```python
from build123d import *

# Parameters (mm, degrees)
F1_DEPTH = 3


with BuildPart() as f1:
    # F0 (on Front) → F1 (new body)
    with BuildSketch(Plane.XZ):
        with BuildLine():
            Line((-2, 0), (0, 0))
            Line((0, 0), (2, 0))
            Line((2, 0), (2, -3))
            Line((2, -3), (8, -3))
            Line((8, -3), (8, 0))
            Line((8, 0), (12, 0))
            Line((12, 0), (12, 30))
            ThreePointArc((12, 30), (8.485281, 38.485281), (0, 42))
            ThreePointArc((0, 42), (-8.485281, 38.485281), (-12, 30))
            Line((-12, 30), (-12, 0))
            Line((-12, 0), (-8, 0))
            Line((-8, 0), (-8, -3))
            Line((-8, -3), (-2, -3))
            Line((-2, -3), (-2, 0))
        make_face()
        with BuildLine():
            ThreePointArc((0, 23.2), (-6.8, 30), (0, 36.8))
            ThreePointArc((0, 36.8), (6.8, 30), (0, 23.2))
        make_face(mode=Mode.SUBTRACT)
    extrude(amount=F1_DEPTH)


solid = f1.part
```
Verification items for the finished model (mm, model axes). A direction names the side the tool comes from. Give positions to 0.01 mm unless a question says otherwise; leave off trailing zeros. Loops run counter-clockwise (first coordinate to the right, second up) from the corner with the lowest first, then second, coordinate; pieces in that order, holes last. Notation, with made-up numbers: M -33,-32 L -3,-32 A30 ccw -3,-2 Z; hole C 82.25,36.25 d7. An arc over 180 degrees is marked long. One line per question, with ' | ' between items.
Item 1: Tool access check on faces 1 (the face through (-10, -1, 0)), 2 (the face through (2, -1, -1)), 3 (the face through (8, -1, -2)). Record the directions out of +Z, -Z, +X, -X, +Y, -Y that give a thin tool (end or side, any length) a straight path to the whole face; none if there is none.
Completed:
face 1: -Z, -X, +Y, -Y | face 2: -Z, +Y, -Y | face 3: -Z, +X, +Y, -Y
Item 2: Section check A-A, the plane z = 32. Record the cut outline in (x, y).
Completed:
outline: M -11.83,-3 L -6.5,-3 L -6.5,0 L -11.83,0 Z; M 6.5,-3 L 11.83,-3 L 11.83,0 L 6.5,0 Z
Item 3: Section check C-C, the plane y = -2.05. Record the cut outline in (x, z).
Completed:
outline: M -12,0 L -8,0 L -8,-3 L -2,-3 L -2,0 L 2,0 L 2,-3 L 8,-3 L 8,0 L 12,0 L 12,30 A12 ccw 0,42 A12 ccw -12,30 Z; hole C 0,30 d13.6
Item 4: Section check D-D, the plane x = -7.5. Record the cut outline in (y, z).
Completed:
outline: M -3,-3 L 0,-3 L 0,39.37 L -3,39.37 Z
Item 5: Section check B-B, the plane x = 4.25. Record the cut outline in (y, z), plus the area to 3 significant figures.
Completed:
outline: M -3,-3 L 0,-3 L 0,24.69 L -3,24.69 Z; M -3,35.31 L 0,35.31 L 0,41.22 L -3,41.22 Z | area: 101 mm^2
Item 6: Depth check by flat-ended pin: P1, Ø1.5, axis at x = 1, y = -1.5, coming from the -Z side; P2, Ø1.5, axis at y = -1.5, z = -1.5, coming from the +X side; P3, Ø1, axis at y = -1.5, z = 33, coming from the -X side; P4, Ø4, axis at x = 5, z = 28.5, coming from the -Y side. Enter the tip coordinate at first touch or a pass-through.
Completed:
P1: stops at z = 0 | P2: stops at x = 8 | P3: stops at x = -11.74 | P4: stops at y = -3
Item 7: Thickness scan on line 1 (X direction, y = -1.5, z = 30); line 2 (X direction, y = -2.35, z = 33.5); line 3 (Z direction, x = 1, y = -1.2). Record the ranges inside material, lowest first. Write a range as [from, to].
Completed:
line 1: x = [-12, -6.8], [6.8, 12] | line 2: x = [-11.48, -5.83], [5.83, 11.48] | line 3: z = [0, 23.27], [36.73, 41.96]
Item 8: Draft check along X on faces 4 (the face through (-12, -1, 15)), 5 (the face through (-2, -1, -2)), 6 (the face through (5, -1, -3)). Enter one of: +X half, -X half, draft (parallel to the pull), parting line (faces both ways), or undercut.
Completed:
face 4: -X half | face 5: undercut | face 6: draft
